CAD build for the part. Positions are in the model's coordinates, mm. A direction names the side the tool comes from. Coordinates: 2 decimals unless noted, no trailing zeros. Write each loop counter-clockwise with the first axis right and the second up, starting at its lowest first coordinate (ties: lowest second). Pieces come first, ordered by that corner, then holes. Notation, with made-up numbers: (32.25, 6) - (55.25, 6) arc R24 ccw to (55.25, 40) - close; hole circle Ø1 at (-13, 88.5). An arc over 180 degrees is marked (long way). Answer in a Markdown table with one row per item. Add a question column.
Q1. Drill centre lines: line 1 along X through (y, z) = (2.3, 17.5); line 2 along Z through (x, y) = (-20.5, 6); line 3 along X through (y, z) = (8.75, 7). Where is each one in solid material? Low to high. Write a range as from..to.
Q2. Band-saw the part on A-A (x = -25). List the corners of the cut face in (y, z), and give its area (3 significant figures).
Q3. Two-plate mould, pull along Y, no slides. Class faces 5 (the flat face through (-5, 25, -3)), 6 (the flat face through (-1, 23, -3)), 7 (the flat face through (-16, 0, -3)), 8 (the cylindrical face through (23, 1, 19)): +Y half, -Y half, draft (parallel to the pull), parting line (faces both ways), or undercut.
Q4. 3-axis set-ups, long thin cutter, end or side, ignore diameter. For faces 1 (the flat face through (-62, 15, -2)), 2 (the flat face through (-16, 14, -42)), 3 (the cylindrical face through (-1.452, 1.756, -42.033)), 4 (the flat face through (-14, 12, -45)): which of +Z, -Z, +X, -X, +Y, -Y reach the whole face in a straight line?
Q5. Band-saw the part on B-B (y = 6). List the corners of the cut face in (x, z), and give its area (3 significant figures).
Q6. Pin check, flat tips, straight feed: pin 1 (8 mm diameter, centred on x = -40, z = -17.5, fed in from +Y); pin 2 (4 mm diameter, centred on x = -25, z = 17.5, fed in from -Y). Stop position of each tip, or through.
Q7. Band-saw the part on D-D (x = -8). List the corners of the cut face in (y, z), and give its area (3 significant figures).
Q8. Band-saw the part on C-C (z = 17.5). List the corners of the cut face in (x, y).
```python
from build123d import *

# Parameters (mm, degrees)
SKETCH1_R           = 2.5
BOSS_EXTRUDE1_DEPTH = 25
SKETCH5_W           = 94
SKETCH5_H           = 79
CUT_EXTRUDE2_DEPTH  = 22
SKETCH7_W           = 85
SKETCH7_H           = 2
BOSS_EXTRUDE4_DEPTH = 66
SKETCH8_R           = 6.7
CUT_EXTRUDE3_DEPTH  = 11
FILLET1_R           = 1.67
SKETCH9_R           = 1.5
SKETCH9_R_2         = 1.2
CUT_EXTRUDE4_DEPTH  = 10


with BuildPart() as part:
    # Sketch1 → Boss-Extrude1 (new body)
    with BuildSketch(Plane(origin=(0, 0, 0), x_dir=(1, 0, 0), z_dir=(0, 1, 0))):
        Polygon((-65, 45), (-65, 37.5), (-65, -32.5), (-65, -40), (35, -40), (35, -32.5), (35, 37.5), (35, 45), align=None)
        with Locations((-25, -17.5)):
            Circle(SKETCH1_R, mode=Mode.SUBTRACT)
        with Locations((25, -17.5)):
            Circle(SKETCH1_R, mode=Mode.SUBTRACT)
        with Locations((-25, 17.5)):
            Circle(SKETCH1_R, mode=Mode.SUBTRACT)
        with Locations((25, 17.5)):
            Circle(SKETCH1_R, mode=Mode.SUBTRACT)
    extrude(amount=BOSS_EXTRUDE1_DEPTH)

    # Sketch5 → Cut-Extrude2 (cut)
    with BuildSketch(Plane(origin=(0, 25, 0), x_dir=(1, 0, 0), z_dir=(0, 1, 0))):
        with Locations((-15, 2.5)):
            Rectangle(SKETCH5_W, SKETCH5_H)
    extrude(amount=-CUT_EXTRUDE2_DEPTH, mode=Mode.SUBTRACT)

    # Sketch7 → Boss-Extrude4 (add)
    with BuildSketch(Plane.ZY.offset(-32)):
        with Locations((-2.5, 24)):
            Rectangle(SKETCH7_W, SKETCH7_H)
    extrude(amount=BOSS_EXTRUDE4_DEPTH)

    # Sketch8 → Cut-Extrude3 (cut)
    with BuildSketch(Plane.XZ):
        with Locations((0, -35.492425409)):
            Circle(SKETCH8_R)
    extrude(amount=-CUT_EXTRUDE3_DEPTH, mode=Mode.SUBTRACT)

    # Fillet1
    fillet1_edges = [part.edges().sort_by_distance(p)[0] for p in [
        (-15, 0, -45),
        (35, 0, -2.5),
        (-15, 0, 40),
        (-65, 0, -2.5),
        (-65, 12.5, -45),
        (35, 12.5, -45),
        (35, 12.5, 40),
        (-65, 12.5, 40),
        (-65, 25, -2.5),
        (32, 3, -2.5),
        (-62, 3, -2.5),
        (-15, 25, 40),
        (35, 25, -2.5),
        (-15, 25, -45),
        (-34, 25, -2.5),
    ]]
    fillet(fillet1_edges, radius=FILLET1_R)

    # Sketch9 → Cut-Extrude4 (cut)
    with BuildSketch(Plane(origin=(0, 3, 0), x_dir=(1, 0, 0), z_dir=(0, 1, 0))):
        with Locations((-48.33, 2.5)):
            Circle(SKETCH9_R)
        with Locations((-48.33, 30.3)):
            Circle(SKETCH9_R_2)
        with Locations((-48.33, -25.3)):
            Circle(SKETCH9_R_2)
    extrude(amount=-CUT_EXTRUDE4_DEPTH, mode=Mode.SUBTRACT)


solid = part.part
```
Checked values:
| question | item | result |
|---|---|---|
| 1 | line 1 | x = -65..-27.5, -22.5..22.5, 27.5..35 |
| 1 | line 2 | z = -45..-42, 37..40 |
| 1 | line 3 | x = -65..-62, 32..35 |
| 2 | outline | (0, -43.33) arc R1.67 ccw to (1.67, -45) - (23.33, -45) arc R1.67 ccw to (25, -43.33) - (25, 38.33) arc R1.67 ccw to (23.33, 40) - (1.67, 40) arc R1.67 ccw to (0, 38.33) - (0, 20) - (3, 20) - (3, 37) - (23, 37) - (23, -42) - (3, -42) - (3, -20) - (0, -20) - close; (0, -15) - (3, -15) - (3, 15) - (0, 15) - close |
| 2 | area | 513 mm² |
| 3 | face 5 | +Y half |
| 3 | face 6 | undercut |
| 3 | face 7 | -Y half |
| 3 | face 8 | draft |
| 4 | face 1 | +Y |
| 4 | face 2 | none |
| 4 | face 3 | -Y |
| 4 | face 4 | -Z, +X, -X, +Y, -Y |
| 5 | outline | (-65, -43.33) arc R1.67 ccw to (-63.33, -45) - (33.33, -45) arc R1.67 ccw to (35, -43.33) - (35, 38.33) arc R1.67 ccw to (33.33, 40) - (-63.33, 40) arc R1.67 ccw to (-65, 38.33) - close; hole (-62, -42) - (-1.59, -42) arc R6.7 ccw to (1.59, -42) - (32, -42) - (32, 37) - (-62, 37) - close |
| 5 | area | 1,070 mm² |
| 6 | pin 1 | stops at y = 3 |
| 6 | pin 2 | stops at y = 23 |
| 7 | outline | (0, -43.33) arc R1.67 ccw to (1.67, -45) - (23.33, -45) arc R1.67 ccw to (25, -43.33) - (25, 38.33) arc R1.67 ccw to (23.33, 40) - (1.67, 40) arc R1.67 ccw to (0, 38.33) - close; hole (3, -42) - (23, -42) - (23, 37) - (3, 37) - close |
| 7 | area | 543 mm² |
| 8 | outline | (-65, 1.67) arc R1.67 ccw to (-63.33, 0) - (-27.5, 0) - (-27.5, 3) - (-60.33, 3) arc R1.67 cw to (-62, 4.67) - (-62, 25) - (-63.33, 25) arc R1.67 ccw to (-65, 23.33) - close; (-34, 23) - (32, 23) - (32, 4.67) arc R1.67 cw to (30.33, 3) - (27.5, 3) - (27.5, 0) - (33.33, 0) arc R1.67 ccw to (35, 1.67) - (35, 23.33) arc R1.67 ccw to (33.33, 25) - (-32.33, 25) arc R1.67 ccw to (-34, 23.33) - close; (-22.5, 0) - (22.5, 0) - (22.5, 3) - (-22.5, 3) - close |
